Geometry check sheet. Reference: the model listing, model coordinates, mm. Round coordinates to 2 decimals unless told otherwise and drop trailing zeros. Loops run counter-clockwise (first coordinate to the right, second up) from the corner with the lowest first, then second, coordinate; pieces in that order, holes last. Notation, with made-up numbers: (-39.75, 45) -> (3.25, 45) arc R20 cw to (3.25, 63) -> close; hole circle Ø1 at (60.5, 59). An arc over 180 degrees is marked (long way). Use one line per item in the form item = value.
from build123d import *

# Parameters (mm, degrees)
SKETCH1_R           = 50.8
BOSS_EXTRUDE1_DEPTH = 381
BOSS_EXTRUDE1_TAPER = 3
DOME1_FACE_RADIUS   = 50.8
DOME1_HEIGHT        = 38.1
SKETCH5_R           = 15.24
CUT_EXTRUDE1_DEPTH  = 254


with BuildPart() as part:
    # Sketch1 → Boss-Extrude1 (new body)
    with BuildSketch(Plane.XY):
        Circle(SKETCH1_R)
    extrude(amount=BOSS_EXTRUDE1_DEPTH, taper=BOSS_EXTRUDE1_TAPER)

    # Dome1: a dome of height H over a round flat face of radius A is a cap of a sphere of radius (A * A + H * H) / (2 * H)
    dome1_r = (DOME1_FACE_RADIUS * DOME1_FACE_RADIUS + DOME1_HEIGHT * DOME1_HEIGHT) / (2 * DOME1_HEIGHT)
    dome1_base = Plane((0, 0, 0), z_dir=(0, 0, -1))
    with Locations(dome1_base.offset(DOME1_HEIGHT - dome1_r)):
        dome1_ball = Sphere(dome1_r, mode=Mode.PRIVATE)
    add(split(dome1_ball, bisect_by=dome1_base, keep=Keep.TOP, mode=Mode.PRIVATE))

    # Sketch5 → Cut-Extrude1 (cut)
    with BuildSketch(Plane.XY.offset(381)):
        Circle(SKETCH5_R)
    extrude(amount=-CUT_EXTRUDE1_DEPTH, mode=Mode.SUBTRACT)


solid = part.part
1. Section check A-A (x = 0). Record the boundary of the cut face in (y, z), then the cut area to 3 significant figures.
Return value:
outline = (-50.8, 0) arc R52.92 ccw to (50.8, 0) -> (30.83, 381) -> (15.24, 381) -> (15.24, 127) -> (-15.24, 127) -> (-15.24, 381) -> (-30.83, 381) -> close
area = 26,200 mm2
2. Material ranges on line 1 along Y through (x, z) = (0, 307); line 2 along Y through (x, z) = (0, 180); line 3 along X through (y, z) = (12.5, 338), recorded low to high.
Return value:
line_1 = -34.71 to -15.24, 15.24 to 34.71
line_2 = -41.37 to -15.24, 15.24 to 41.37
line_3 = -30.63 to -8.72, 8.72 to 30.63
3. Section check D-D (z = 9.5). Record the boundary of the cut face in (x, y), then the cut area to 3 significant figures.
Return value:
outline = circle Ø100.6 at (0, 0)
area = 7,950 mm2
4. Mould release check, pull along X, two halves, no side actions. Record for faces 1 (the conical face through (37.575, -15.579, 193.167)), 2 (the flat face through (6.4, 14.1, 381)), 3 (the flat face through (0, 0, 127)): released by +X, released by -X, zero draft, split by the parting line, or undercut.
Return value:
face_1 = split by the parting line
face_2 = zero draft
face_3 = undercut
5. Gauge pin test, flat ends, axial feed: pin 1 (1 mm diameter, centred on x = -10, y = 5.5, fed in from -Z); pin 2 (1.5 mm diameter, centred on x = -36, z = 308.5, fed in from -Y); pin 3 (6 mm diameter, centred on y = -28, z = 220, fed in from +X); pin 4 (9 mm diameter, centred on x = -7, y = 7, fed in from +Z). Record the tip position at first contact, or that the pin passes through.
Return value:
pin_1 = -36.96
pin_2 = through
pin_3 = 30.29
pin_4 = 127
6. Section check C-C (z = 218). Record the boundary of the cut face in (x, y), then the cut area to 3 significant figures.
Return value:
outline = circle Ø78.75 at (0, 0); hole circle Ø30.48 at (0, 0)
area = 4,140 mm2
